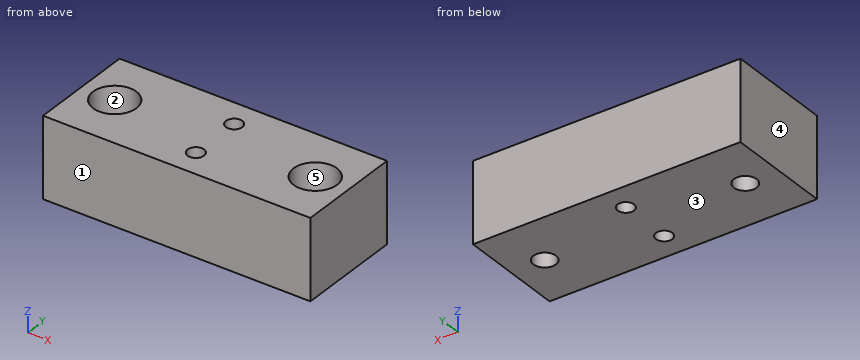
Autodesk Inventor part; units mm, degrees
ref_plane "YZ Plane" through (0, 0, 0) normal (1, 0, 0) x (0, 1, 0)
ref_plane "XZ Plane" through (0, 0, 0) normal (0, 1, 0) x (-1, 0, 0)
ref_plane "XY Plane" through (0, 0, 0) normal (0, 0, 1) x (1, 0, 0)
sketch "Skizze1" plane through (0, 0, 0) normal (0, 0, 1) x (1, 0, 0)
  line L0 (0, 0) -> (40, 0)
  line L1 (40, 0) -> (40, 16)
  line L2 (40, 16) -> (0, 16)
  line L3 (0, 16) -> (0, 0)
  dimension "d0" = 16
  dimension "d1" = 40
extrude "Extrusion1" add sketch "Skizze1" along normal blind 12
sketch "Skizze2" plane through (0, 0, 12) normal (0, 0, 1) x (1, 0, 0)
  line L0 (40, 0) -> (0, 0)
  line L1 (0, 16) -> (40, 16)
  line L2 (20, 16) -> (20, 0)
  point P0 (20, 12)
  point P1 (20, 4)
  dimension "d4" = 4
  dimension "d5" = 8
hole "Bohrung1" at (20, 12, 12) at (20, 4, 12) direction (0, 0, -1) diameter 2.459 end through all
sketch "Skizze3" plane through (0, 0, 12) normal (0, 0, 1) x (1, 0, 0)
  line L0 (0, 0) -> (0, 16)
  line L1 (40, 0) -> (0, 0)
  line L2 (40, 16) -> (40, 0)
  line L3 (0, 16) -> (40, 16)
  line L4 (0, 8) -> (40, 8)
  line L5 (20, 16) -> (20, 0)
  point P0 (5, 8)
  point P1 (35, 8)
  dimension "d13" = 30
hole "Bohrung2" at (5, 8, 12) at (35, 8, 12) direction (0, 0, -1) diameter 3.4 end through all counterbore diameter 6.5 counterbore depth 5
properties part number "13_0204_069"
Check sheet for the modelled part. Datum: model origin and axes. Units: mm. Face numbers are marked on the shaded views. A direction names the side the tool comes from. Round coordinates to 2 decimals unless told otherwise and drop trailing zeros. Loops run counter-clockwise (first coordinate to the right, second up) from the corner with the lowest first, then second, coordinate; pieces in that order, holes last. Notation, with made-up numbers: (-28, 83) -> (11, 83) arc R21 cw to (11, 105) -> close; hole circle Ø11 at (62, 63). An arc over 180 degrees is marked (long way). Put each result on its own line as item: value. Start each with the question number.
1. Draft check along Y on the marked faces 1, 2 and 3. Enter one of: +Y half, -Y half, draft (parallel to the pull), parting line (faces both ways), or undercut.
2. Access from +Z, -Z, +X, -X, +Y, -Y to the whole of each face (thin tool, end or side, straight path). Record for the marked faces 4 and 5.
3. Section check C-C (x = 20). Enter the section's corners in (y, z), plus the area to 3 significant figures.
4. Section check D-D (y = 8). Enter the section's corners in (x, z).
5. Section check B-B (z = 7.75). Enter the section's corners in (x, y), plus the area to 3 significant figures.
6. Gauge pin test, flat ends, axial feed: pin 1 (2 mm diameter, centred on x = 20, y = 4, fed in from +Z); pin 2 (5 mm diameter, centred on x = 35, y = 8, fed in from +Z). Record the tip position at first contact, or that the pin passes through.
7. Section check A-A (y = 12). Enter the section's corners in (x, z).
8. Scan lines: probe 1 along X at (y, z) = (8.25, 11.25); probe 2 along X at (y, z) = (8, 5); probe 3 along Y at (x, z) = (35, 5.75). Record each from-to range of solid material in increasing order.
Findings:
1. face 1: -Y half
1. face 2: undercut
1. face 3: draft
2. face 4: +Z, -Z, -X, +Y, -Y
2. face 5: +Z
3. outline: (0, 0) -> (2.77, 0) -> (2.77, 12) -> (0, 12) -> close; (5.23, 0) -> (10.77, 0) -> (10.77, 12) -> (5.23, 12) -> close; (13.23, 0) -> (16, 0) -> (16, 12) -> (13.23, 12) -> close
3. area: 133 mm^2
4. outline: (0, 0) -> (3.3, 0) -> (3.3, 7) -> (1.75, 7) -> (1.75, 12) -> (0, 12) -> close; (6.7, 0) -> (33.3, 0) -> (33.3, 7) -> (31.75, 7) -> (31.75, 12) -> (8.25, 12) -> (8.25, 7) -> (6.7, 7) -> close; (36.7, 0) -> (40, 0) -> (40, 12) -> (38.25, 12) -> (38.25, 7) -> (36.7, 7) -> close
5. outline: (0, 0) -> (40, 0) -> (40, 16) -> (0, 16) -> close; hole circle Ø6.5 at (5, 8); hole circle Ø2.46 at (20, 4); hole circle Ø2.46 at (20, 12); hole circle Ø6.5 at (35, 8)
5. area: 564 mm^2
6. pin 1: passes through
6. pin 2: stops at z = 7
7. outline: (0, 0) -> (18.77, 0) -> (18.77, 12) -> (0, 12) -> close; (21.23, 0) -> (40, 0) -> (40, 12) -> (21.23, 12) -> close
8. probe 1: x = 0 to 1.76, 8.24 to 31.76, 38.24 to 40
8. probe 2: x = 0 to 3.3, 6.7 to 33.3, 36.7 to 40
8. probe 3: y = 0 to 6.3, 9.7 to 16
